For this review, take the finished solid that the model builds, in its own axes (mm). Coordinates: 2 decimals unless noted, no trailing zeros. Loops run counter-clockwise (first coordinate to the right, second up) from the corner with the lowest first, then second, coordinate; pieces in that order, holes last. Notation, with made-up numbers: M -4,52 L 1,52 A26 cw 1,72 Z; hole C 26,-40 d10. An arc over 180 degrees is marked long. Write item = value, one per line.
from build123d import *

# Parameters (mm, degrees)
SKETCH2_W           = 115
SKETCH2_H           = 40
BOSS_EXTRUDE1_DEPTH = 60
CUT_EXTRUDE1_DEPTH  = 60
SKETCH4_R           = 10
CUT_EXTRUDE2_DEPTH  = 60


with BuildPart() as part:
    # Sketch2 → Boss-Extrude1 (new body)
    with BuildSketch(Plane.XY):
        with Locations((-2.12962963, 23.505291005)):
            Rectangle(SKETCH2_W, SKETCH2_H)
    extrude(amount=BOSS_EXTRUDE1_DEPTH)

    # Sketch3 → Cut-Extrude1 (cut)
    with BuildSketch(Plane(origin=(0, 43.505291005, 0), x_dir=(1, 0, 0), z_dir=(0, 1, 0))):
        with BuildLine():
            Line((-59.62962963, -30), (-24.62962963, -30))
            ThreePointArc((-24.62962963, -30), (-2.12962963, -7.5), (20.37037037, -30))
            Line((20.37037037, -30), (55.37037037, -30))
            Line((55.37037037, -30), (55.37037037, -60))
            Line((55.37037037, -60), (-59.62962963, -60))
            Line((-59.62962963, -60), (-59.62962963, -30))
        make_face()
    extrude(amount=-CUT_EXTRUDE1_DEPTH, mode=Mode.SUBTRACT)

    # Sketch4 → Cut-Extrude2 (cut)
    with BuildSketch(Plane.XY.offset(30)):
        with Locations((-42.12962963, 23.505291005)):
            Circle(SKETCH4_R)
        with Locations((37.87037037, 23.505291005)):
            Circle(SKETCH4_R)
    extrude(amount=-CUT_EXTRUDE2_DEPTH, mode=Mode.SUBTRACT)


solid = part.part
Q1. Add section C-C (z = 26). Write out the cut boundary in (x, y), and give its area (3 significant figures).
Solved:
outline = M -59.63,3.51 L -24.27,3.51 L -24.27,43.51 L -59.63,43.51 Z; M 20.01,3.51 L 55.37,3.51 L 55.37,43.51 L 20.01,43.51 Z; hole C -42.13,23.51 d20; hole C 37.87,23.51 d20
area = 2,200 mm²
Q2. Add section D-D (z = 2). Write out the cut boundary in (x, y).
Solved:
outline = M -59.63,3.51 L 55.37,3.51 L 55.37,43.51 L -59.63,43.51 Z; hole C -42.13,23.51 d20; hole C 37.87,23.51 d20
Q3. For line 1 along X through (y, z) = (19, 22); line 2 along X through (y, z) = (19, 1); line 3 along X through (y, z) = (21.5, 18), list the stretches that pass through material, from the lowest coordinate up.
Solved:
line_1 = -59.63 to -51.06, -33.2 to -23.16, 18.9 to 28.94, 46.8 to 55.37
line_2 = -59.63 to -51.06, -33.2 to 28.94, 46.8 to 55.37
line_3 = -59.63 to -51.93, -32.33 to -21.16, 16.9 to 28.07, 47.67 to 55.37
Q4. Add section A-A (z = 10). Write out the cut boundary in (x, y).
Solved:
outline = M -59.63,3.51 L -12.44,3.51 L -12.44,43.51 L -59.63,43.51 Z; M 8.18,3.51 L 55.37,3.51 L 55.37,43.51 L 8.18,43.51 Z; hole C -42.13,23.51 d20; hole C 37.87,23.51 d20
Q5. Add section B-B (y = 32). Write out the cut boundary in (x, z).
Solved:
outline = M -59.63,0 L -47.41,0 L -47.41,30 L -59.63,30 Z; M -36.85,0 L 32.59,0 L 32.59,30 L 20.37,30 A22.5 cw -24.63,30 L -36.85,30 Z; M 43.15,0 L 55.37,0 L 55.37,30 L 43.15,30 Z
Q6. Draft analysis for pull direction X (two halves, no side actions). For faces 1 (the face through (-44.297, 13.743, 15.21)), 2 (the face through (-59.63, 23, 15)), 3 (the face through (-46, 33, 30)), state which applies: +X half, -X half, draft (parallel to the pull), parting line (faces both ways), or undercut.
Solved:
face_1 = undercut
face_2 = -X half
face_3 = draft
